Verification items for the finished model (mm, model axes). A direction names the side the tool comes from. Round coordinates to 2 decimals unless told otherwise and drop trailing zeros. Write each loop counter-clockwise with the first axis right and the second up, starting at its lowest first coordinate (ties: lowest second). Pieces come first, ordered by that corner, then holes. Notation, with made-up numbers: (53, -24) - (92, -24) arc R34 cw to (92, 6) - close; hole circle Ø7 at (18.25, -27). An arc over 180 degrees is marked (long way). Answer as a JSON object with one key per item and string values. Group by question number.
1) Section check A-A (y = 12). Enter the section's corners in (x, z).
2) Section check B-B (y = -5.5). Enter the section's corners in (x, z) (3 decimals), then the cut area to 3 significant figures.
3) Mould release check, pull along Y, two halves, no side actions. Record for faces 4 (the flat face through (25.267, 15.226, 70.137)), 5 (the cylindrical face through (7.55, 0.813, 63.667)), 6 (the cylindrical face through (-22.978, 1.011, 20.288)), 7 (the flat face through (16, -13, 13)): +Y half, -Y half, draft (parallel to the pull), parting line (faces both ways), or undercut.
4) Thickness scan on line 1 (Y direction, x = 0, z = 8); line 2 (Y direction, x = 0, z = 27.5); line 3 (Y direction, x = -3, z = 5.5). Record the ranges inside material, lowest first.
5) Set-up check for faces 1 (the flat face through (23.97, 5.88, 72.38)), 2 (the cylindrical face through (-2.799, 21.317, 6.409)), 3 (the flat face through (6, -18, 0)): record each of +Z, -Z, +X, -X, +Y, -Y from which the full face is reachable in a straight line by a thin tool's end or side.
6) Go/stop test with flat-tipped pins: pin 1 Ø8 at (x, y) = (36, -13.5) entering from -Z; pin 2 Ø4 at (y, z) = (4.5, 10.5) entering from +X; pin 3 Ø1 at (x, z) = (29, 32) entering from -Y. Record where each tip stops, or that it passes through.
```python
from build123d import *

# Parameters (mm, degrees)
F1_R     = 23
F1_R_2   = 21.5
F1_R_3   = 20
F1_R_4   = 18.5
F3_R     = 21.35
F3_R_2   = 20.15
F4_DEPTH = 13
F5_DEPTH = 13


with BuildPart() as f2:
    # F2: sweep along a path in F0
    with BuildLine(Plane.XZ) as f2_path:
        Line((0, 0), (0, 37.9670113325))
        Line((0, 37.9670113325), (32.880303367, 56.9504633325))
    # F1 (on Top) → F2 (sweep)
    with BuildSketch(Plane.XY):
        Circle(F1_R)
        Circle(F1_R_2, mode=Mode.SUBTRACT)
        Circle(F1_R_2)
        Circle(F1_R_3, mode=Mode.SUBTRACT)
        Circle(F1_R_3)
        Circle(F1_R_4, mode=Mode.SUBTRACT)
    sweep(path=f2_path.line, transition=Transition.RIGHT)

    # F3 (on face) → F4 (join)
    with BuildSketch(Plane(origin=(49.3205015269, 0, 28.4752048331), x_dir=(0, 1, 0), z_dir=(0.8660254038, 0, 0.5))):
        with Locations((0, 32.8803963197)):
            Circle(F3_R)
        with Locations((0, 32.8803963197)):
            Circle(F3_R_2, mode=Mode.SUBTRACT)
    extrude(amount=F4_DEPTH)

    # F1 (on Top) → F5 (cut)
    with BuildSketch(Plane.XY):
        Circle(F1_R_2)
        Circle(F1_R_3, mode=Mode.SUBTRACT)
    extrude(amount=F5_DEPTH, mode=Mode.SUBTRACT)


solid = f2.part
```
Returned:
{
 "1": {"outline": "(-19.62, 0) - (-17.84, 0) - (-17.84, 13) - (-16, 13) - (-16, 0) - (-14.08, 0) - (-14.08, 46.1) - (25.84, 69.14) - (24.79, 70.97) - (36.05, 77.47) - (35.31, 78.74) - (24.05, 72.24) - (23.07, 73.94) - (-19.62, 49.3) - close; (14.08, 0) - (16, 0) - (16, 13) - (17.84, 13) - (17.84, 0) - (19.62, 0) - (19.62, 26.64) - (42.69, 39.96) - (41.71, 41.66) - (52.97, 48.16) - (52.23, 49.43) - (40.97, 42.93) - (39.92, 44.76) - (14.08, 29.84) - close"},
 "2": {"outline": "(-22.333, 0) - (-20.785, 0) - (-20.785, 13) - (-19.229, 13) - (-19.229, 0) - (-17.664, 0) - (-17.664, 48.165) - (24.049, 72.248) - (23.188, 73.738) - (34.446, 80.238) - (33.824, 81.316) - (22.566, 74.816) - (21.714, 76.291) - (-22.333, 50.861) - close; (17.664, 0) - (19.229, 0) - (19.229, 13) - (20.785, 13) - (20.785, 0) - (22.333, 0) - (22.333, 25.073) - (44.047, 37.61) - (43.195, 39.085) - (54.453, 45.585) - (53.831, 46.663) - (42.573, 40.163) - (41.712, 41.653) - (17.664, 27.769) - close", "area": "701 mm2"},
 "3": {"face 4": "draft", "face 5": "undercut", "face 6": "parting line", "face 7": "undercut"},
 "4": {"line 1": "-23 to -21.5, -20 to -18.5, 18.5 to 20, 21.5 to 23", "line 2": "-23 to -18.5, 18.5 to 23", "line 3": "-22.8 to -21.29, -19.77 to -18.26, 18.26 to 19.77, 21.29 to 22.8"},
 "5": {"face 1": "none", "face 2": "-Z", "face 3": "-Z, +X, -X, +Y, -Y"},
 "6": {"pin 1": "z = 33.59", "pin 2": "x = 22.86", "pin 3": "y = -12.71"}
}
